from build123d import *

# Parameters (mm, degrees)
SKETCH_1_W                   = 62
SKETCH_1_H                   = 37
EXTRUDE_1_DEPTH              = 13
HOLE_WIZARD_M5_1_D           = 5.8
HOLE_WIZARD_M5_1_CBORE_D     = 10
HOLE_WIZARD_M5_1_CBORE_DEPTH = 5
HOLE_WIZARD_M4_3_D           = 4.8
HOLE_WIZARD_M4_3_CBORE_D     = 8
HOLE_WIZARD_M4_3_CBORE_DEPTH = 4


with BuildPart() as part:
    # 草图1 → 凸台-拉伸1 (new body)
    with BuildSketch(Plane.XY):
        with Locations((31, 18.5)):
            Rectangle(SKETCH_1_W, SKETCH_1_H)
    extrude(amount=EXTRUDE_1_DEPTH)

    # M5 六角凹头螺钉的柱形沉头孔1 (through all)
    with Locations(Plane(origin=(0, 0, 0), x_dir=(-1, 0, 0), z_dir=(0, 0, -1))):
        with Locations((-7, 11), (-7, 29), (-55, 11), (-55, 29)):
            CounterBoreHole(HOLE_WIZARD_M5_1_D / 2, HOLE_WIZARD_M5_1_CBORE_D / 2, HOLE_WIZARD_M5_1_CBORE_DEPTH)

    # M4 六角凹头螺钉的柱形沉头孔3 (through all)
    with Locations(Plane.XY.offset(13)):
        with Locations((39, 16), (23, 16), (23, 31), (39, 31)):
            CounterBoreHole(HOLE_WIZARD_M4_3_D / 2, HOLE_WIZARD_M4_3_CBORE_D / 2, HOLE_WIZARD_M4_3_CBORE_DEPTH)


solid = part.part
Input: part model. Units: mm. Frame: model coordinates. A direction names the side the tool comes from. Coordinates: 2 decimals unless noted, no trailing zeros. Loops run counter-clockwise (first coordinate to the right, second up) from the corner with the lowest first, then second, coordinate; pieces in that order, holes last.
Q1. Set-up query: faces 1 (the face through (22.479, 34.966, 11.028)), 2 (the face through (4.8, 26.8, 5)), 3 (the face through (57.766, 29.871, 9.056)). Return all of +Z, -Z, +X, -X, +Y, -Y with unobstructed straight access to the full face (end or side cutting, diameter ignored); none if empty.
Q2. Cut plane B-B (z = 1.5). Give the number of separate pieces and of enclosed holes in the cut face, then the cut area to 3 significant figures.
Q3. Cut plane C-C (x = 23). Output: boundary loops of the cut face in (y, z).
Q4. Cut plane A-A (x = 7). Output: boundary loops of the cut face in (y, z).
Q5. Contact query for flat-ended pins moving along their axis: pin 1 (4 mm diameter, centred on x = 22, y = 17, fed in from +Z); pin 2 (3 mm diameter, centred on x = 9.5, y = 31, fed in from -Z). Output: stop coordinate, or through.
Q6. Material intervals for line 1 (Y direction, x = 23, z = 10.9); line 2 (Y direction, x = 7, z = 11.75); line 3 (X direction, y = 17.5, z = 7), sorted ascending.
Q7. Draft query along X for faces 4 (the face through (4.8, 8.8, 5)), 5 (the face through (31, 0, 6)), 6 (the face through (23.52, 28.657, 4.437)), 7 (the face through (0, 18, 6)). Return one class per face: +X half, -X half, draft (parallel to the pull), parting line (faces both ways), or undercut.
Working result:
1. face 1: +Z
1. face 2: -Z
1. face 3: +Z, -Z
2. separate pieces: 1
2. enclosed holes: 8
2. area: 1,910 mm2
3. outline: (0, 0) - (13.6, 0) - (13.6, 9) - (12, 9) - (12, 13) - (0, 13) - close; (18.4, 0) - (28.6, 0) - (28.6, 9) - (27, 9) - (27, 13) - (20, 13) - (20, 9) - (18.4, 9) - close; (33.4, 0) - (37, 0) - (37, 13) - (35, 13) - (35, 9) - (33.4, 9) - close
4. outline: (0, 0) - (6, 0) - (6, 5) - (8.1, 5) - (8.1, 13) - (0, 13) - close; (13.9, 5) - (16, 5) - (16, 0) - (24, 0) - (24, 5) - (26.1, 5) - (26.1, 13) - (13.9, 13) - close; (31.9, 5) - (34, 5) - (34, 0) - (37, 0) - (37, 13) - (31.9, 13) - close
5. pin 1: stops at z = 9
5. pin 2: stops at z = 5
6. line 1: y = 0 to 12, 20 to 27, 35 to 37
6. line 2: y = 0 to 8.1, 13.9 to 26.1, 31.9 to 37
6. line 3: x = 0 to 21.13, 24.87 to 37.13, 40.87 to 62
7. face 4: undercut
7. face 5: draft
7. face 6: undercut
7. face 7: -X half
